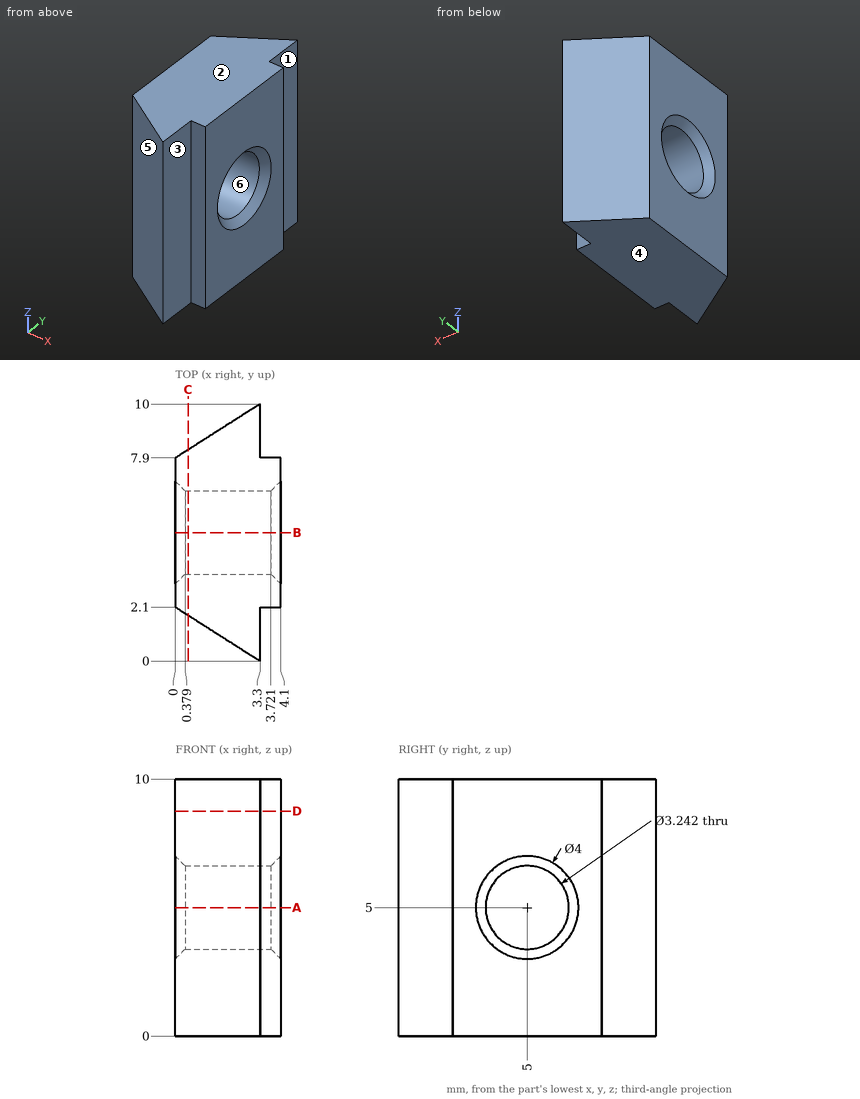
Here's the drawing with two shaded views (mm, measured from the low corner). I have some questions. A direction names the side the tool comes from. Give positions to 0.01 mm unless a question says otherwise; leave off trailing zeros. Loops run counter-clockwise (first coordinate to the right, second up) from the corner with the lowest first, then second, coordinate; pieces in that order, holes last. Notation, with made-up numbers: M 82.5,73 L 136.5,73 A21 ccw 136.5,92 Z; hole C -4.75,-16.5 d3. An arc over 180 degrees is marked long. One line per item, written item: value.
1) On a 3-axis mill with a long thin cutter (end or side, diameter ignored), from which of +Z, -Z, +X, -X, +Y, -Y can I reach the whole of each face in a straight line? I mean the marked faces 1, 2 and 3. Say none if no direction works.
Geometry check:
face 1: +Z, -Z, +X, +Y
face 2: +Z, +X, -X, +Y, -Y
face 3: +Z, -Z, +X, -Y
2) Imagine slicing it at D-D on z = 8.75. Write out the boundary of the cut face in (x, y).
Geometry check:
outline: M 0,2.1 L 3.3,0 L 3.3,2.1 L 4.1,2.1 L 4.1,7.9 L 3.3,7.9 L 3.3,10 L 0,7.9 Z
3) Imagine slicing it at A-A on z = 5. Write out the boundary of the cut face in (x, y), and give its area (3 significant figures).
Geometry check:
outline: M 0,2.1 L 3.3,0 L 3.3,2.1 L 4.1,2.1 L 4.1,3 L 3.72,3.38 L 0.38,3.38 L 0,3 Z; M 0,7 L 0.38,6.62 L 3.72,6.62 L 4.1,7 L 4.1,7.9 L 3.3,7.9 L 3.3,10 L 0,7.9 Z
area: 17.1 mm²
4) Imagine slicing it at C-C on x = 0.5. Write out the boundary of the cut face in (y, z), and give its area (3 significant figures).
Geometry check:
outline: M 1.78,0 L 8.22,0 L 8.22,10 L 1.78,10 Z; hole C 5,5 d3.24
area: 56.1 mm²
5) Please list where these lines run through material, in increasing order: line 1 (Z direction, x = 2.6, y = 5); line 2 (Y direction, x = 1.8, z = 4.75); line 3 (Y direction, x = 3.85, z = 8).
Geometry check:
line 1: z = 0 to 3.38, 6.62 to 10
line 2: y = 0.95 to 3.4, 6.6 to 9.05
line 3: y = 2.1 to 7.9
6) Imagine slicing it at B-B on y = 5. Write out the boundary of the cut face in (x, z).
Geometry check:
outline: M 0,0 L 4.1,0 L 4.1,3 L 3.72,3.38 L 0.38,3.38 L 0,3 Z; M 0,7 L 0.38,6.62 L 3.72,6.62 L 4.1,7 L 4.1,10 L 0,10 Z
7) Thinking about a two-plate mould opening in Y: for the marked faces 4, 5 and 6, which applies, +Y half, -Y half, draft (parallel to the pull), parting line (faces both ways), or undercut?
Geometry check:
face 4: draft
face 5: -Y half
face 6: undercut
8) I'm going to push flat-ended pins straight in: pin 1 (1 mm diameter, centred on x = 2.5, z = 3.5, fed in from -Y); pin 2 (2.5 mm diameter, centred on y = 5, z = 5, fed in from +X); pin 3 (0.9 mm diameter, centred on x = 4, z = 7.5, fed in from -Y); pin 4 (1.7 mm diameter, centred on y = 9, z = 7.5, fed in from +X). Where does each tip first touch, or does it pass through?
Geometry check:
pin 1: stops at y = 0.19
pin 2: passes through
pin 3: stops at y = 2.1
pin 4: stops at x = 3.3
